Autodesk Inventor part; units mm, degrees
ref_plane "YZ Plane" through (0, 0, 0) normal (1, 0, 0) x (0, 1, 0)
ref_plane "XZ Plane" through (0, 0, 0) normal (0, 1, 0) x (-1, 0, 0)
ref_plane "XY Plane" through (0, 0, 0) normal (0, 0, 1) x (1, 0, 0)
sketch "Sketch1" plane through (0, 0, 0) normal (0, 1, 0) x (-1, 0, 0)
  line L0 (0, 0) -> (0, -152.4)
  line L1 (0, 0) -> (0, 5.08)
  line L2 (0, 5.08) -> (1.27, 5.08)
  line L3 (1.27, 5.08) -> (1.27, 0)
  line L4 (1.27, 0) -> (0, 0)
  line L5 (0, 0) -> (0, -4.826)
  line L6 (0, -4.826) -> (1.397, -4.826)
  line L7 (1.397, -4.826) -> (1.397, 0)
  line L8 (1.397, 0) -> (1.27, 0)
  line L9 (0, 0) -> (0, -7.62)
  line L10 (4.445, -7.62) -> (2.54, 0)
  line L11 (4.445, -152.4) -> (4.445, -7.62)
  line L12 (2.54, 0) -> (2.2936, -0.0616)
  line L13 (2.2936, -0.0616) -> (4.1986, -7.6816)
  line L14 (4.1986, -7.6816) -> (4.1986, -152.4)
  line L15 (4.1986, -152.4) -> (4.445, -152.4)
  line L16 (1.397, -4.826) -> (4.1986, -7.6816)
  line L17 (0, -152.4) -> (3.81, -152.4)
  line L18 (3.81, -152.4) -> (3.81, -146.304)
  line L19 (3.81, -146.304) -> (0, -146.304)
  line L20 (3.81, -146.304) -> (4.445, -146.304)
  dimension "d0" = 152.4
  dimension "d1" = 5.08
  dimension "d2" = 1.27
  dimension "d3" = 4.826
  dimension "d4" = 1.397
  dimension "d5" = 2.54
  dimension "d6" = 7.62
  dimension "d7" = 4.445
  dimension "d8" = 4.445
  dimension "d9" = 0.254
  dimension "d10" = 3.81
  dimension "d11" = 6.096
  dimension "d21" = 0.2464
revolve "Revolution1" add sketch "Sketch1" angle 360 about axis through (0, 0, 0) along (0, 0, -1)
sketch "Sketch2" plane through (0, 0, -152.4) normal (0, 0, -1) x (-1, 0, 0)
  line L0 (0, 0) -> (0, -0.762)
  line L1 (0, -0.762) -> (3.733, -0.762)
  circle A0 centre (0, 0) radius 3.81
  line L2 (0, -0.762) -> (-3.733, -0.762)
  line L3 (0, 0) -> (0, 0.762)
  line L4 (0, 0.762) -> (3.733, 0.762)
  line L5 (0, 0.762) -> (-3.733, 0.762)
  dimension "d13" = 0.762
  dimension "d14" = 0.762
extrude "Extrusion1" add sketch "Sketch2" along normal blind 8.89 contours L3 L4 A0 L1 L0 | L0 L2 A0 L5 L3
fillet "Fillet1" radius 1.016 4 edges at (-3.81, 0, -161.29) (3.81, 0, -161.29) (0, 0.762, -152.4) (0, -0.762, -152.4)
chamfer "Chamfer1" distance 1.016 distance2 0.508 1 edges at (1.27, 0, 5.08) measured on face at (-1.2659, -0.1022, 1.6933)
sketch "Sketch3" plane through (-3.733, -0.762, -153.416) normal (0, -1, 0) x (1, 0, 0)
  point P0 (3.733, 153.416)
properties part number "Pencil Body"
Design review of the part built by this model. Coordinates are the model's own, in mm. A direction names the side the tool comes from. Round coordinates to 2 decimals unless told otherwise and drop trailing zeros. Write each loop counter-clockwise with the first axis right and the second up, starting at its lowest first coordinate (ties: lowest second). Pieces come first, ordered by that corner, then holes. Notation, with made-up numbers: (77, -39.75) -> (111, -39.75) arc R20 cw to (111, -15.75) -> close; hole circle Ø3 at (-40, 77). An arc over 180 degrees is marked (long way). One line per item, written item: value. Start each with the question number.
Q1. Add section A-A (z = -108). Give the boundary of the cut face in (x, y) (3 decimals), then the cut area to 3 significant figures.
Q2. Tool access review of faces 4 (the face through (0.96, 4.34, -79)), 5 (the face through (0.661, -2.975, -3.078)), 6 (the face through (1.11, 0.85, -2.38)), 7 (the face through (-4.005, 1.261, -149.395)), 8 (the face through (0, -0.762, -157)): name each direction out of +Z, -Z, +X, -X, +Y, -Y from which nothing blocks a thin tool from reaching the whole face with its end or side.
Q3. To check wall thickness, follow probe 1 along Y at (x, z) = (0, -147.25) (3 decimals); probe 2 along X at (y, z) = (1.25, -146.5); probe 3 along X at (y, z) = (1.5, -58). State the ranges of each line that lie inside material, in increasing order.
Q4. Insertion check: P1, Ø3, axis at x = -3, z = -138, coming from the -Y side; P2, Ø2, axis at x = 1.5, z = -135.5, coming from the -Y side; P3, Ø1, axis at y = -2.5, z = -24, coming from the +X side. Each pin has a flat end and moves straight along its axis. Give the tip position at first contact, or say it passes through.
Q5. The part is to be moulded in two halves that separate along X. For faces 1 (the face through (-1.5, 0.472, -5.005)), 2 (the face through (0.17, 1.26, 2)), 3 (the face through (0, 0.762, -157)), say which applies: pulls with the +X half, pulls with the -X half, needs draft (parallel to the pull), parting line crosses it, or undercut.
Response:
1. outline: circle Ø8.89 at (0, 0)
1. area: 62.1 mm^2
2. face 4: +Z, -Z
2. face 5: none
2. face 6: +Z
2. face 7: -Z
2. face 8: -Z, +X, -X, -Y
3. probe 1: y = -4.445 to -4.199, -3.81 to 3.81, 4.199 to 4.445
3. probe 2: x = -4.27 to -4.01, -3.6 to 3.6, 4.01 to 4.27
3. probe 3: x = -4.18 to 4.18
4. P1: stops at y = -4.18
4. P2: stops at y = -4.42
4. P3: stops at x = 3.97
5. face 1: undercut
5. face 2: parting line crosses it
5. face 3: needs draft
